Drawing for the job (mm, zero at the part's lowest x, y, z). Round coordinates to 2 decimals unless told otherwise and drop trailing zeros. Order: outer loops, then holes, each group sorted by start corner. A loop starts at its lowest first (then second) coordinate and runs counter-clockwise, first axis right, second up. Notation, with made-up numbers: (63.5, 32) - (69.5, 32) arc R20 cw to (69.5, 37) - close; hole circle Ø7 at (76.25, 9.25). An arc over 180 degrees is marked (long way). Answer as a JSON object with one key per item and string values.
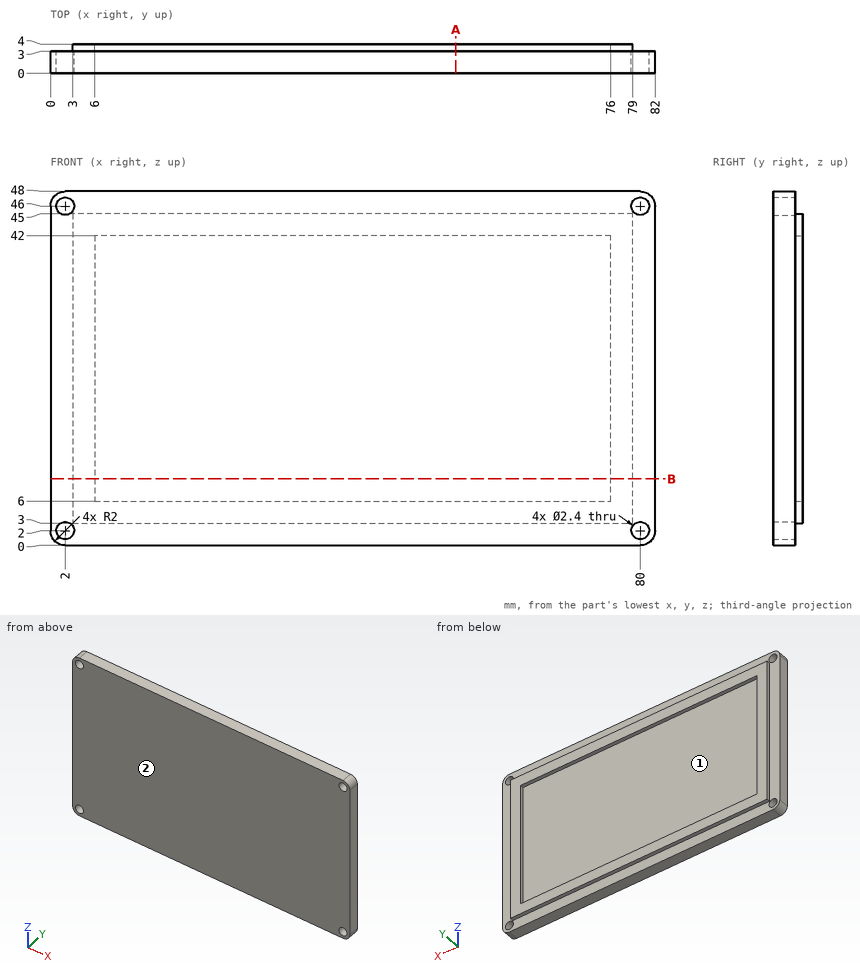
Item 1: Probe L1, parallel to X at y = 1.3, z = 46; L2, parallel to Z at x = 2, y = 2; L3, parallel to Z at x = 34, y = 3.1. List the from-to ranges inside material, lowest first. Write a range as from..to.
Taken from the geometry:
{"L1": "0..0.8, 3.2..78.8, 81.2..82", "L2": "0..0.8, 3.2..44.8, 47.2..48", "L3": "3..6, 42..45"}
Item 2: Drop flat-ended pins along their axis: P1, Ø3, axis at x = 80, z = 2, coming from the -Y side; P2, Ø0.5, axis at x = 43, y = 3.5, coming from the -Z side; P3, Ø0.5, axis at x = 55.5, y = 3.5, coming from the +Z side; P4, Ø0.5, axis at y = 3.5, z = 19, coming from the +X side. Give the stop position or say it passes through.
Taken from the geometry:
{"P1": "y = 0", "P2": "z = 3", "P3": "z = 45", "P4": "x = 79"}
Item 3: Two-plate mould, pull along Z, no slides. Class the marked faces 1 and 2: pulls with the +Z half, pulls with the -Z half, needs draft (parallel to the pull), parting line crosses it, or undercut.
Taken from the geometry:
{"face 1": "undercut", "face 2": "needs draft"}
Item 4: Cut at B-B (z = 9). Write the cut outline in (x, y).
Taken from the geometry:
{"outline": "(0, 0) - (82, 0) - (82, 3) - (79, 3) - (79, 4) - (76, 4) - (76, 3) - (6, 3) - (6, 4) - (3, 4) - (3, 3) - (0, 3) - close"}
Item 5: Cut at A-A (x = 55). Write the cut outline in (y, z).
Taken from the geometry:
{"outline": "(0, 0) - (3, 0) - (3, 3) - (4, 3) - (4, 6) - (3, 6) - (3, 42) - (4, 42) - (4, 45) - (3, 45) - (3, 48) - (0, 48) - close"}
